from build123d import *

# Parameters (mm, degrees)
F0_R     = 3.02
F1_DEPTH = 5
F3_DEPTH = 5


with BuildPart() as f1:
    # F0 (on Top) → F1 (new body)
    with BuildSketch(Plane.XY):
        Circle(F0_R)
    extrude(amount=F1_DEPTH)

    # F2 (on face) → F3 (cut)
    with BuildSketch(Plane.XY.offset(5)):
        with BuildLine():
            ThreePointArc((-2.4270044643, 1.2280266), (-2.3555890983, -1.36), (-0.15, -2.7158608212))
            Line((-0.15, -2.7158608212), (-0.15, -0.0866025404))
            Line((-0.15, -0.0866025404), (-2.4270044643, 1.2280266))
        make_face()
        with BuildLine():
            Line((0, 0.1732050808), (2.2770044643, 1.4878342212))
            ThreePointArc((2.2770044643, 1.4878342212), (0, 2.72), (-2.2770044643, 1.4878342212))
            Line((-2.2770044643, 1.4878342212), (0, 0.1732050808))
        make_face()
        with BuildLine():
            ThreePointArc((0.15, -2.7158608212), (1.9756517912, -1.8695453993), (2.72, 0))
            ThreePointArc((2.72, 0), (2.6457373398, 0.6312479137), (2.4270044643, 1.2280266))
            Line((2.4270044643, 1.2280266), (0.15, -0.0866025404))
            Line((0.15, -0.0866025404), (0.15, -2.7158608212))
        make_face()
    extrude(amount=-F3_DEPTH, mode=Mode.SUBTRACT)


solid = f1.part
Could you check a few things on this model? Use its own coordinates, in mm. A direction names the side the tool comes from. Give positions to 0.01 mm unless a question says otherwise; leave off trailing zeros. Order: outer loops, then holes, each group sorted by start corner. A loop starts at its lowest first (then second) coordinate and runs counter-clockwise, first axis right, second up.
Item 1: For faces 1 (the face through (0, 0, 0)), 2 (the face through (0.04, 2.72, 2.54)), which set-ups out of +Z, -Z, +X, -X, +Y, -Y let a thin tool reach every point of the face, with its end or its side?
Item 2: If we section it at D-D, the plane x = 2: Write out the boundary of the cut face in (y, z).
Item 3: If we section it at C-C, the plane y = 1.75: Write out the boundary of the cut face in (x, z).
Item 4: If we section it at B-B, the plane z = 2.2: Write out the boundary of the cut face in (x, y).
Item 5: If we mould it in two halves opening along X, with no side actions, what happens to faces 3 (the face through (0, 0, 5)), 4 (the face through (-0.393, 2.994, 2.465)), 5 (the face through (-1.27, 0.56, 2.54))? For each: pulls with the +X half, pulls with the -X half, needs draft (parallel to the pull), parting line crosses it, or undercut.
Item 6: I need wall thicknesses on line 1 (Y direction, x = 0.5, z = 2.3); line 2 (X direction, y = 0.75, z = 2.7); line 3 (Y direction, x = -0.75, z = 1.6). Which ranges of each line are inside material? Lowest first, please.
Item 7: I'm going to push flat-ended pins straight in: pin 1 (0.8 mm diameter, centred on y = -1.5, z = 3.5, fed in from +X); pin 2 (1 mm diameter, centred on x = 2, z = 2, fed in from +Y); pin 3 (1.3 mm diameter, centred on y = -2, z = 3, fed in from -X). Where does each tip first touch, or does it pass through?
Item 8: If we section it at A-A, the plane y = -2.5: Write out the boundary of the cut face in (x, z).
Values:
1. face 1: -Z, +X, -X, +Y, -Y
1. face 2: +Z, -Z
2. outline: (-2.26, 0) - (-1.84, 0) - (-1.84, 5) - (-2.26, 5) - close; (0.98, 0) - (1.33, 0) - (1.33, 5) - (0.98, 5) - close; (1.84, 0) - (2.26, 0) - (2.26, 5) - (1.84, 5) - close
3. outline: (-2.46, 0) - (-2.08, 0) - (-2.08, 5) - (-2.46, 5) - close; (2.08, 0) - (2.46, 0) - (2.46, 5) - (2.08, 5) - close
4. outline: circle Ø6.04 at (0, 0); hole (-2.43, 1.23) arc R2.72 ccw to (-0.15, -2.72) - (-0.15, -0.09) - close; hole (-2.28, 1.49) - (0, 0.17) - (2.28, 1.49) arc R2.72 ccw to start; hole (0.15, -2.72) arc R2.72 ccw to (2.43, 1.23) - (0.15, -0.09) - close
5. face 3: needs draft
5. face 4: parting line crosses it
5. face 5: undercut
6. line 1: y = -2.98 to -2.67, 0.12 to 0.46, 2.67 to 2.98
6. line 2: x = -2.93 to -2.61, -1.6 to -1, 1 to 1.6, 2.61 to 2.93
6. line 3: y = -2.93 to -2.61, 0.26 to 0.61, 2.61 to 2.93
7. pin 1: stops at x = 2.81
7. pin 2: stops at y = 2.62
7. pin 3: stops at x = -2.7
8. outline: (-1.69, 0) - (-1.07, 0) - (-1.07, 5) - (-1.69, 5) - close; (-0.15, 0) - (0.15, 0) - (0.15, 5) - (-0.15, 5) - close; (1.07, 0) - (1.69, 0) - (1.69, 5) - (1.07, 5) - close
